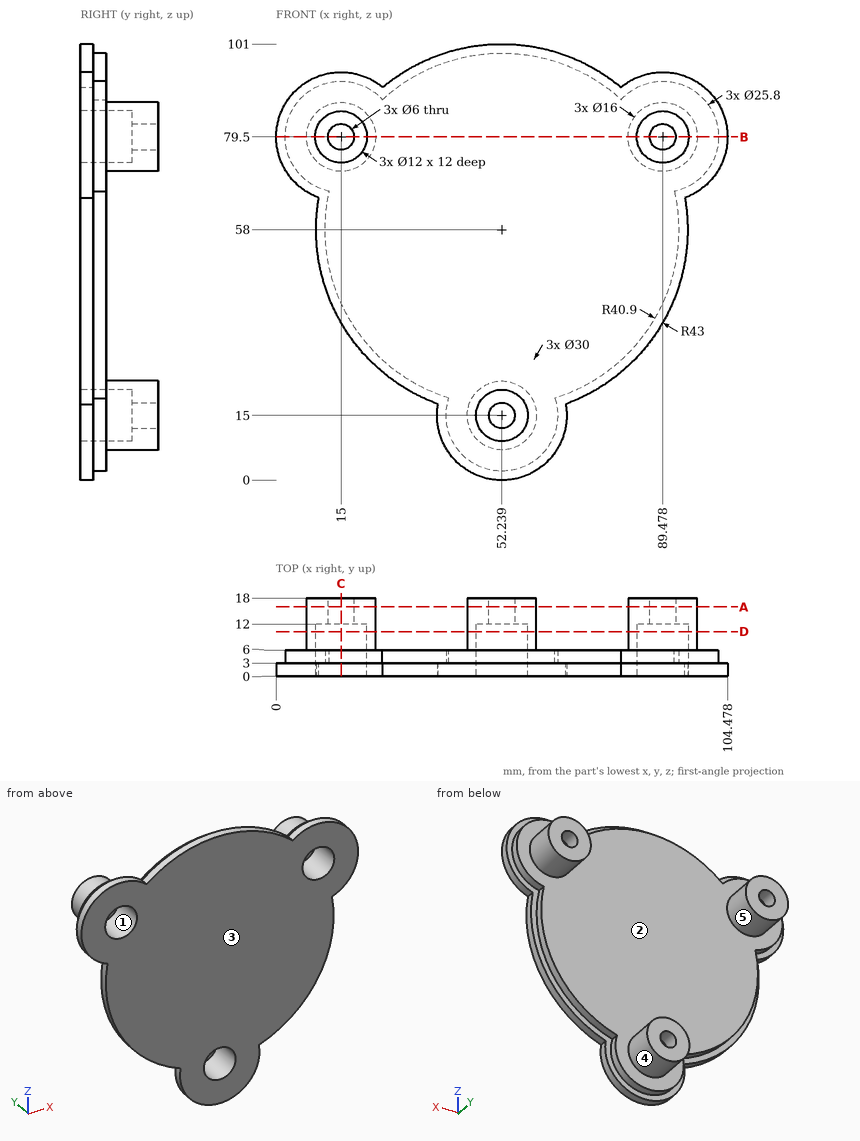
Geometry check sheet. Reference: drawing and pictorial views, mm from the part's lowest x, y, z. A direction names the side the tool comes from. Give positions to 0.01 mm unless a question says otherwise; leave off trailing zeros. Write each loop counter-clockwise with the first axis right and the second up, starting at its lowest first coordinate (ties: lowest second). Pieces come first, ordered by that corner, then holes. Notation, with made-up numbers: (-25.75, 40.25) - (2.25, 40.25) arc R9 ccw to (2.25, 53.25) - close; hole circle Ø2 at (12, 46.25). An arc over 180 degrees is marked (long way). Put each result on its own line as item: value.
Q1. Section check D-D on y = 10.25. Record the cut outline in (x, z).
Result:
outline: circle Ø16 at (15, 79.5); circle Ø16 at (52.24, 15); circle Ø16 at (89.48, 79.5); hole circle Ø12 at (15, 79.5); hole circle Ø12 at (52.24, 15); hole circle Ø12 at (89.48, 79.5)
Q2. Section check C-C on x = 15. Record the cut outline in (y, z), and give its area (3 significant figures).
Result:
outline: (0, 36.5) - (3, 36.5) - (3, 41.09) - (6, 41.09) - (6, 71.5) - (18, 71.5) - (18, 76.5) - (12, 76.5) - (12, 73.5) - (0, 73.5) - close; (0, 85.5) - (12, 85.5) - (12, 82.5) - (18, 82.5) - (18, 87.5) - (6, 87.5) - (6, 92.4) - (3, 92.4) - (3, 94.5) - (0, 94.5) - close
area: 340 mm2
Q3. Section check B-B on z = 79.5. Count the separate pieces of the cut face and the enclosed holes in it, and give its area (3 significant figures).
Result:
separate pieces: 3
enclosed holes: 0
area: 638 mm2
Q4. Set-up check for the marked faces 1 and 2: record each of +Z, -Z, +X, -X, +Y, -Y from which the full face is reachable in a straight line by a thin tool's end or side.
Result:
face 1: -Y
face 2: +Y
Q5. Section check A-A on y = 16. Record the cut outline in (x, z), and give its area (3 significant figures).
Result:
outline: circle Ø16 at (15, 79.5); circle Ø16 at (52.24, 15); circle Ø16 at (89.48, 79.5); hole circle Ø6 at (15, 79.5); hole circle Ø6 at (52.24, 15); hole circle Ø6 at (89.48, 79.5)
area: 518 mm2
Q6. Mould release check, pull along X, two halves, no side actions. Record for the marked faces 3, 4 and 5: released by +X, released by -X, zero draft, split by the parting line, or undercut.
Result:
face 3: zero draft
face 4: split by the parting line
face 5: undercut
Q7. Depth check by flat-ended pin: P1, Ø3.5, axis at x = 88, z = 80, coming from the -Y side; P2, Ø1.5, axis at y = 7.5, z = 51.5, coming from the +X side; P3, Ø5, axis at y = 3.5, z = 66.5, coming from the +X side; P4, Ø3, axis at y = 3.5, z = 11.5, coming from the +X side. Enter the tip coordinate at first touch or a pass-through.
Result:
P1: y = 12
P2: through
P3: x = 100.14
P4: x = 67.09
Q8. Scan lines: probe 1 along X at (y, z) = (15.2, 79.5); probe 2 along Z at (x, y) = (15, 13.35); probe 3 along X at (y, z) = (8.5, 79.5). Record each from-to range of solid material in increasing order. Write a range as from..to.
Result:
probe 1: 7..12, 18..23, 81.48..86.48, 92.48..97.48
probe 2: 71.5..76.5, 82.5..87.5
probe 3: 7..9, 21..23, 81.48..83.48, 95.48..97.48
